Source: three-view drawing plus pictorial views. Frame: mm from the lowest corner of the part. A direction names the side the tool comes from. Round coordinates to 2 decimals unless told otherwise and drop trailing zeros. Loops run counter-clockwise (first coordinate to the right, second up) from the corner with the lowest first, then second, coordinate; pieces in that order, holes last. Notation, with made-up numbers: (47, 29) -> (60, 29) arc R26 cw to (60, 66) -> close; hole circle Ø3 at (50, 0.5). An arc over 180 degrees is marked (long way). Answer in a Markdown table with one row per item.
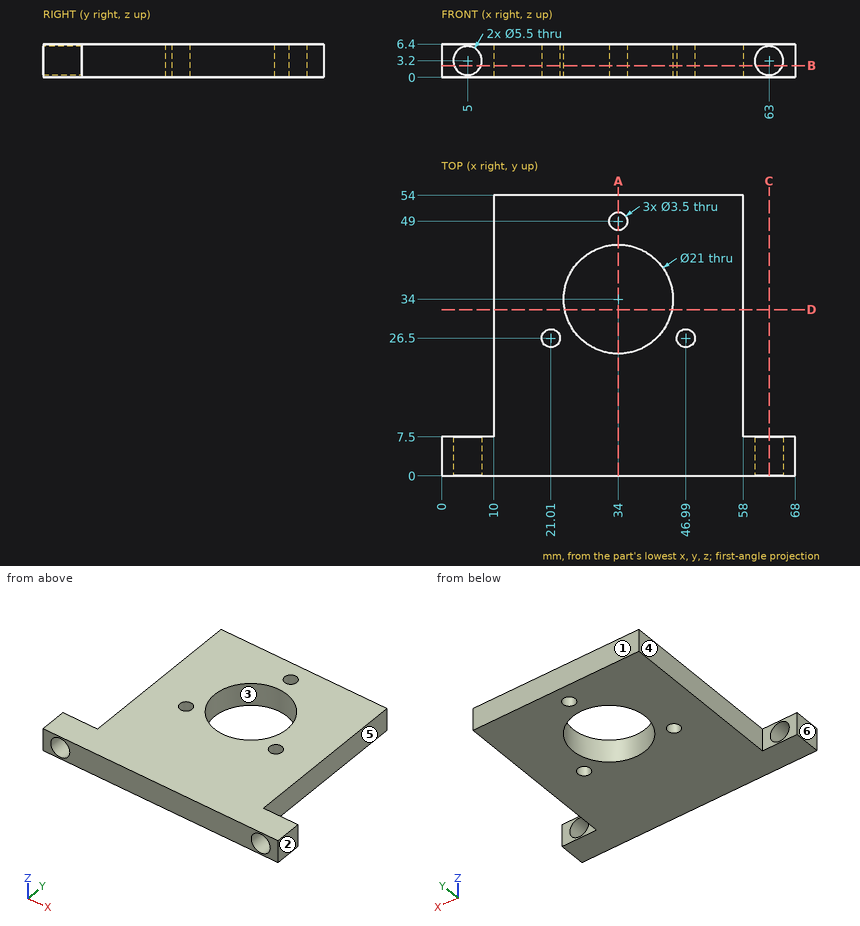
Item 1: Cut plane A-A (x = 34). Output: boundary loops of the cut face in (y, z), then the cut area to 3 significant figures.
Answer:
| item | result |
|---|---|
| outline | (0, 0) -> (23.5, 0) -> (23.5, 6.4) -> (0, 6.4) -> close; (44.5, 0) -> (47.25, 0) -> (47.25, 6.4) -> (44.5, 6.4) -> close; (50.75, 0) -> (54, 0) -> (54, 6.4) -> (50.75, 6.4) -> close |
| area | 189 mm² |
Item 2: Reachability of the marked faces 5 and 6 from +Z, -Z, +X, -X, +Y, -Y: full face, straight path, thin tool, end or side. Return the list, or none.
Answer:
| item | result |
|---|---|
| face 5 | +Z, -Z, +X, +Y |
| face 6 | +Z, -Z, -X, +Y, -Y |
Item 3: Cut plane C-C (x = 63). Output: boundary loops of the cut face in (y, z).
Answer:
| item | result |
|---|---|
| outline | (0, 0) -> (7.5, 0) -> (7.5, 0.45) -> (0, 0.45) -> close; (0, 5.95) -> (7.5, 5.95) -> (7.5, 6.4) -> (0, 6.4) -> close |
Item 4: Pin query (flat end, axial travel): pin 1 Ø2 at (y, z) = (29.5, 3) entering from -X. Return the tip coordinate at first contact, or that it passes through.
Answer:
| item | result |
|---|---|
| pin 1 | stops at x = 10 |
Item 5: Line query: probe 1 along X at (y, z) = (27.5, 1) (1 decimal); probe 2 along X at (y, z) = (46.5, 4.5); probe 3 along Y at (x, z) = (26, 3). Output: solid intervals per line, ascending. Write a range as [from, to].
Answer:
| item | result |
|---|---|
| probe 1 | x = [10, 19.6], [22.4, 25.8], [42.2, 45.6], [48.4, 58] |
| probe 2 | x = [10, 58] |
| probe 3 | y = [0, 27.2], [40.8, 54] |
Item 6: Cut plane D-D (y = 32). Output: boundary loops of the cut face in (x, z), then the cut area to 3 significant figures.
Answer:
| item | result |
|---|---|
| outline | (10, 0) -> (23.69, 0) -> (23.69, 6.4) -> (10, 6.4) -> close; (44.31, 0) -> (58, 0) -> (58, 6.4) -> (44.31, 6.4) -> close |
| area | 175 mm² |
Item 7: Cut plane B-B (z = 2.25). Count the separate pieces of the cut face and the enclosed holes in it, then the cut area to 3 significant figures.
Answer:
| item | result |
|---|---|
| separate pieces | 3 |
| enclosed holes | 4 |
| area | 2,290 mm² |
Item 8: Draft query along X for the marked faces 1, 2, 3 and 4. Return one class per face: pulls with the +X half, pulls with the -X half, needs draft (parallel to the pull), parting line crosses it, or undercut.
Answer:
| item | result |
|---|---|
| face 1 | needs draft |
| face 2 | pulls with the +X half |
| face 3 | undercut |
| face 4 | pulls with the -X half |
